Can you work these out from the model? Positions are in its coordinate system, mm. Coordinates: 2 decimals unless noted, no trailing zeros. Return JSON: item names as keys, results as strings. Group by question number.
1) If we mould it in two halves opening along X, with no side actions, what happens to faces 1 (the face through (0.806, -74.535, 0.789)), 2 (the face through (-1, 1, 0))? For each: pulls with the +X half, pulls with the -X half, needs draft (parallel to the pull), parting line crosses it, or undercut.
2) Imagine slicing it at A-A (z = 0.5). Give the number of separate pieces and of enclosed holes in the cut face, and give its area (3 significant figures).
3) If I drill on line 1 along Y through (x, z) = (16.5, 0.65); line 2 along Y through (x, z) = (-9, 0.65); line 3 along X through (y, z) = (-22.8, 0.75), over which ranges is the centre line in solid material (lowest first)?
```python
from build123d import *

# Parameters (mm, degrees)
SKETCH1_W                    = 82.5
SKETCH1_H                    = 156.7
SKETCH1_R                    = 0.8
SKETCH1_R_2                  = 1.5
BASE_SHAPE_DEPTH             = 1.6
PCB_CORNER_FILLETS_R         = 1
SKETCH6_R                    = 1.5
SOLAR_CONNECTOR_CUTOUT_DEPTH = 1.6
SOLAR_HOLE_FILLETS_R         = 0.5
M2_CLEARANCE_HOLE1_D         = 2.4
M2_CLEARANCE_HOLE1_DEPTH     = 1.6
SKETCH10_W                   = 1.75
SKETCH10_H                   = 2.4
SCREW_SLOTS_DEPTH            = 89.559838527


with BuildPart() as part:
    # Sketch1 → Base shape (new body)
    with BuildSketch(Plane.XY):
        Rectangle(SKETCH1_W, SKETCH1_H)
        with Locations((-39.5, 58.6)):
            Circle(SKETCH1_R, mode=Mode.SUBTRACT)
        with Locations((-39.5, 28.6)):
            Circle(SKETCH1_R, mode=Mode.SUBTRACT)
        with Locations((-39.5, 0)):
            Circle(SKETCH1_R, mode=Mode.SUBTRACT)
        with Locations((-39.5, -28.6)):
            Circle(SKETCH1_R, mode=Mode.SUBTRACT)
        with Locations((-39.5, -58.6)):
            Circle(SKETCH1_R, mode=Mode.SUBTRACT)
        with Locations((0, -75.8)):
            Circle(SKETCH1_R_2, mode=Mode.SUBTRACT)
        with Locations((39.5, -58.6)):
            Circle(SKETCH1_R, mode=Mode.SUBTRACT)
        with Locations((39.5, -28.6)):
            Circle(SKETCH1_R, mode=Mode.SUBTRACT)
        with Locations((39.5, 0)):
            Circle(SKETCH1_R, mode=Mode.SUBTRACT)
        with Locations((39.5, 28.6)):
            Circle(SKETCH1_R, mode=Mode.SUBTRACT)
        with Locations((39.5, 58.6)):
            Circle(SKETCH1_R, mode=Mode.SUBTRACT)
        with Locations((-16.5, 22.8)):
            Circle(SKETCH1_R, mode=Mode.SUBTRACT)
        with Locations((-16.5, -22.8)):
            Circle(SKETCH1_R, mode=Mode.SUBTRACT)
        with Locations((16.5, -22.8)):
            Circle(SKETCH1_R, mode=Mode.SUBTRACT)
        with Locations((16.5, 22.8)):
            Circle(SKETCH1_R, mode=Mode.SUBTRACT)
        with Locations((0, 75.8)):
            Circle(SKETCH1_R_2, mode=Mode.SUBTRACT)
    extrude(amount=BASE_SHAPE_DEPTH)

    # PCB corner fillets
    pcb_corner_fillets_edges = [part.edges().sort_by_distance(p)[0] for p in [
        (41.25, -78.35, 0.8),
        (-41.25, -78.35, 0.8),
        (-41.25, 78.35, 0.8),
        (41.25, 78.35, 0.8),
    ]]
    fillet(pcb_corner_fillets_edges, radius=PCB_CORNER_FILLETS_R)

    # Sketch6 → Solar connector cutout (cut)
    with BuildSketch(Plane(origin=(0, 0, 0), x_dir=(-1, 0, 0), z_dir=(0, 0, -1))):
        with Locations(Location((0, 75.8, 0), (0, 0, 180))):
            Circle(SKETCH6_R)
        with BuildLine():
            Line((9.5, 76.5), (3, 76.5))
            Line((3, 76.5), (3, 73))
            Line((3, 73), (-3, 73))
            Line((-3, 73), (-3, 76.5))
            Line((-3, 76.5), (-9.5, 76.5))
            ThreePointArc((-9.5, 76.5), (-10, 76), (-9.5, 75.5))
            Line((-9.5, 75.5), (-6.2, 75.5))
            Line((-6.2, 75.5), (-6.2, 68.2))
            Line((-6.2, 68.2), (6.2, 68.2))
            Line((6.2, 68.2), (6.2, 75.5))
            Line((6.2, 75.5), (9.5, 75.5))
            ThreePointArc((9.5, 75.5), (10, 76), (9.5, 76.5))
        make_face()
    solar_connector_cutout = extrude(amount=-SOLAR_CONNECTOR_CUTOUT_DEPTH, mode=Mode.SUBTRACT)

    # Mirror solar cutout: Solar connector cutout across plane
    add(solar_connector_cutout.mirror(Plane.ZX), mode=Mode.SUBTRACT)

    # Solar Hole fillets
    solar_hole_fillets_edges = [part.edges().sort_by_distance(p)[0] for p in [
        (-3, 76.5, 0.8),
        (-3, 73, 0.8),
        (3, 73, 0.8),
        (3, 76.5, 0.8),
        (6.2, 75.5, 0.8),
        (6.2, 68.2, 0.8),
        (-6.2, 68.2, 0.8),
        (-6.2, 75.5, 0.8),
        (-3, -73, 0.8),
        (3, -73, 0.8),
        (6.2, -75.5, 0.8),
        (6.2, -68.2, 0.8),
        (-6.2, -68.2, 0.8),
        (-6.2, -75.5, 0.8),
    ]]
    fillet(solar_hole_fillets_edges, radius=SOLAR_HOLE_FILLETS_R)

    # M2 Clearance Hole1
    with Locations(Plane(origin=(39.5, 58.6, 0), x_dir=(-1, 0, 0), z_dir=(0, 0, -1))):
        with Locations((0, 0), (0, -30), (23, -35.8), (56, -35.8), (79, -30), (79, 0), (79, -58.6), (0, -58.6), (23, -81.4), (56, -81.4), (79, -87.2), (0, -87.2), (0, -117.2), (79, -117.2)):
            Hole(M2_CLEARANCE_HOLE1_D / 2, depth=M2_CLEARANCE_HOLE1_DEPTH)

    # Sketch10 → Screw Slots (cut, through all)
    with BuildSketch(Plane(origin=(0, 0, 0), x_dir=(-1, 0, 0), z_dir=(0, 0, -1))):
        with Locations((40.375, 58.6)):
            Rectangle(SKETCH10_W, SKETCH10_H)
        with Locations((40.375, 28.6)):
            Rectangle(SKETCH10_W, SKETCH10_H)
        with Locations((40.375, 0)):
            Rectangle(SKETCH10_W, SKETCH10_H)
        with Locations((40.375, -28.6)):
            Rectangle(SKETCH10_W, SKETCH10_H)
        with Locations((40.375, -58.6)):
            Rectangle(SKETCH10_W, SKETCH10_H)
        with Locations((-40.375, -58.6)):
            Rectangle(SKETCH10_W, SKETCH10_H)
        with Locations((-40.375, -28.6)):
            Rectangle(SKETCH10_W, SKETCH10_H)
        with Locations((-40.375, 0)):
            Rectangle(SKETCH10_W, SKETCH10_H)
        with Locations((-40.375, 28.6)):
            Rectangle(SKETCH10_W, SKETCH10_H)
        with Locations((-40.375, 58.6)):
            Rectangle(SKETCH10_W, SKETCH10_H)
    extrude(amount=-SCREW_SLOTS_DEPTH, mode=Mode.SUBTRACT)


solid = part.part
```
Calculated:
{
 "1": {"face 1": "undercut", "face 2": "needs draft"},
 "2": {"separate pieces": "1", "enclosed holes": "8", "area": "12,700 mm2"},
 "3": {"line 1": "-78.35 to -24, -21.6 to 21.6, 24 to 78.35", "line 2": "-78.35 to -76.5, -75.5 to 75.5, 76.5 to 78.35", "line 3": "-41.25 to -17.7, -15.3 to 15.3, 17.7 to 41.25"}
}
